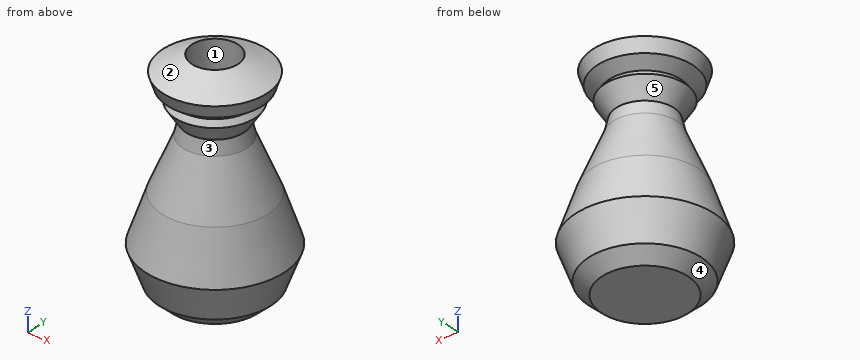
```python
from build123d import *

# Parameters (mm, degrees)
F2_R     = 14.973683
F3_DEPTH = 88.392
F4_DEPTH = 68.58


with BuildPart() as f1:
    # F0 (on Front) → F1 (revolve)
    with BuildSketch(Plane.XZ):
        Polygon((0, -79.605266), (0, 70.394734), (-33.717105, 52.467106), (-30.921052, 44.078944), (-23.355263, 38.486842), (-26.014588, 34.888929), (-18.749999, 23.519738), (-20.723683, 14.967105), (-34.539474, -18.421052), (-44.901316, -49.01316), (-36.513158, -71.710529), (-27.960526, -79.605266), align=None)
    revolve(axis=Axis((0, 0, -4.605266), (0, 0, -1)))

    # F2 (on Top) → F3 (cut)
    with BuildSketch(Plane.XY):
        Circle(F2_R)
    extrude(amount=F3_DEPTH, mode=Mode.SUBTRACT)

    # F2 (on Top) → F4 (cut)
    with BuildSketch(Plane.XY):
        Circle(F2_R)
    extrude(amount=-F4_DEPTH, mode=Mode.SUBTRACT)


solid = f1.part
```
Source: CAD feature listing. Evaluate the final solid. Frame: model axes, mm. Face numbers are marked on the shaded views. A direction names the side the tool comes from. Give positions to 0.01 mm unless a question says otherwise; leave off trailing zeros. Write each loop counter-clockwise with the first axis right and the second up, starting at its lowest first coordinate (ties: lowest second). Pieces come first, ordered by that corner, then holes. Notation, with made-up numbers: (34.25, 60.5) - (60.25, 60.5) arc R21 cw to (60.25, 89.5) - close; hole circle Ø1 at (75.25, 65.5). An arc over 180 degrees is marked (long way). One line per item, written item: value. Start each with the question number.
Q1. Material intervals for probe 1 along Z at (x, y) = (23.5, 3); probe 2 along Y at (x, z) = (0, -26); probe 3 along Z at (x, y) = (28, 0.5), sorted ascending. Write a range as from..to.
Q2. Section query B-B, the plane z = -25.5. Return the cut outline in (x, y).
Q3. Section query D-D, the plane z = -4. Return the cut outline in (x, y), then the cut area to 3 significant figures.
Q4. Set-up query: the marked faces 4 and 5. Return all of +Z, -Z, +X, -X, +Y, -Y with unobstructed straight access to the full face (end or side cutting, diameter ignored); none if empty.
Q5. Section query A-A, the plane y = 0. Return the cut outline in (x, z), then the cut area to 3 significant figures.
Q6. First-contact query: pin 1 Ø12 at (x, z) = (-10, -10) entering from -Y; pin 2 Ø10 at (x, z) = (34.5, -13.5) entering from -Y; pin 3 Ø10 at (x, z) = (-7, -25) entering from +Y. Flat tips, straight axial feed; report the tip coordinate or a pass-through.
Q7. Draft query along Z for the marked faces 1, 2 and 3. Return one class per face: +Z half, -Z half, draft (parallel to the pull), parting line (faces both ways), or undercut.
Answer:
1. probe 1: z = -79.61..7.8, 31.25..38.03, 38.73..57.8
1. probe 2: y = -37.11..-14.97, 14.97..37.11
1. probe 3: z = -79.56..-2.63, 41.92..55.5
2. outline: circle Ø73.87 at (0, 0); hole circle Ø29.95 at (0, 0)
3. outline: circle Ø57.14 at (0, 0); hole circle Ø29.95 at (0, 0)
3. area: 1,860 mm2
4. face 4: -Z
4. face 5: none
5. outline: (-44.9, -49.01) - (-36.51, -71.71) - (-27.96, -79.61) - (27.96, -79.61) - (36.51, -71.71) - (44.9, -49.01) - (34.54, -18.42) - (20.72, 14.97) - (18.75, 23.52) - (26.01, 34.89) - (23.36, 38.49) - (30.92, 44.08) - (33.72, 52.47) - (14.97, 62.43) - (14.97, -68.58) - (-14.97, -68.58) - (-14.97, 62.43) - (-33.72, 52.47) - (-30.92, 44.08) - (-23.36, 38.49) - (-26.01, 34.89) - (-18.75, 23.52) - (-20.72, 14.97) - (-34.54, -18.42) - close
5. area: 5,060 mm2
6. pin 1: stops at y = -32.46
6. pin 2: stops at y = -14.7
6. pin 3: stops at y = 37.99
7. face 1: draft
7. face 2: +Z half
7. face 3: undercut
